```python
from build123d import *

# Parameters (mm, degrees)
SKETCH_1_W          = 15
SKETCH_1_H          = 15
SKETCH_1_W_2        = 13
SKETCH_1_H_2        = 13
EXTRUDE_1_DEPTH     = 37
SKETCH_2_R          = 1.45
CUT_EXTRUDE_1_DEPTH = 41.623269194
SKETCH_3_R          = 1.45
CUT_EXTRUDE_2_DEPTH = 41.623269194


with BuildPart() as part:
    # 草图1 → 凸台-拉伸1 (new body)
    with BuildSketch(Plane(origin=(0, 0, 0), x_dir=(0, 0, -1), z_dir=(1, 0, 0))):
        Rectangle(SKETCH_1_W, SKETCH_1_H)
        Rectangle(SKETCH_1_W_2, SKETCH_1_H_2, mode=Mode.SUBTRACT)
    extrude(amount=EXTRUDE_1_DEPTH)

    # 草图2 → 切除-拉伸1 (cut, through all)
    with BuildSketch(Plane(origin=(0, 0, -7.5), x_dir=(-1, 0, 0), z_dir=(0, 0, -1))):
        with Locations((-11, 0)):
            Circle(SKETCH_2_R)
        with Locations((-26, 0)):
            Circle(SKETCH_2_R)
    extrude(amount=-CUT_EXTRUDE_1_DEPTH, mode=Mode.SUBTRACT)

    # 草图3 → 切除-拉伸2 (cut, through all)
    with BuildSketch(Plane(origin=(0, 7.5, 0), x_dir=(1, 0, 0), z_dir=(0, 1, 0))):
        with Locations(Location((10, 0, 0), (0, 0, 270))):
            Circle(SKETCH_3_R)
        with Locations(Location((30, 0, 0), (0, 0, 270))):
            Circle(SKETCH_3_R)
        with Locations(Location((20, 0, 0), (0, 0, 270))):
            Circle(SKETCH_3_R)
    extrude(amount=-CUT_EXTRUDE_2_DEPTH, mode=Mode.SUBTRACT)


solid = part.part
```
Geometry check sheet. Reference: the model listing, model coordinates, mm. A direction names the side the tool comes from. Give positions to 0.01 mm unless a question says otherwise; leave off trailing zeros. Write each loop counter-clockwise with the first axis right and the second up, starting at its lowest first coordinate (ties: lowest second). Pieces come first, ordered by that corner, then holes.
1) Section check C-C, the plane x = 10. Record the boundary of the cut face in (y, z).
2) Material ranges on L1, parallel to X at y = 7.05, z = 0; L2, parallel to Z at x = 26, y = 2.75, recorded low to high.
3) Section check B-B, the plane x = 26. Record the boundary of the cut face in (y, z), and give its area (3 significant figures).
4) Section check D-D, the plane y = -2. Record the boundary of the cut face in (x, z).
5) Access from +Z, -Z, +X, -X, +Y, -Y to the whole of each face (thin tool, end or side, straight path). Record for faces 4 (the flat face through (18, 6.5, 0)), 5 (the cylindrical face through (24.62, 0.44, -7.01)).
6) Release check for a two-part mould opening along Y. For faces 1 (the cylindrical face through (24.62, 0.44, 6.99)), 2 (the flat face through (18, 0, 7.5)), 3 (the flat face through (18, 7.5, 0)) record: pulls with the +Y half, pulls with the -Y half, needs draft (parallel to the pull), parting line crosses it, or undercut.
7) Section check A-A, the plane z = -1. State how many separate pieces and enclosed holes the cut face has, and give its area (3 significant figures).
Computed:
1. outline: (-7.5, -7.5) - (-1.05, -7.5) - (-1.05, -6.5) - (-6.5, -6.5) - (-6.5, -1.45) - (-7.5, -1.45) - close; (-7.5, 1.45) - (-6.5, 1.45) - (-6.5, 6.5) - (-1.05, 6.5) - (-1.05, 7.5) - (-7.5, 7.5) - close; (1.05, -7.5) - (7.5, -7.5) - (7.5, -1.45) - (6.5, -1.45) - (6.5, -6.5) - (1.05, -6.5) - close; (1.05, 6.5) - (6.5, 6.5) - (6.5, 1.45) - (7.5, 1.45) - (7.5, 7.5) - (1.05, 7.5) - close
2. L1: x = 0 to 8.55, 11.45 to 18.55, 21.45 to 28.55, 31.45 to 37
2. L2: z = -7.5 to -6.5, 6.5 to 7.5
3. outline: (-7.5, -7.5) - (-1.45, -7.5) - (-1.45, -6.5) - (-6.5, -6.5) - (-6.5, 6.5) - (-1.45, 6.5) - (-1.45, 7.5) - (-7.5, 7.5) - close; (1.45, -7.5) - (7.5, -7.5) - (7.5, 7.5) - (1.45, 7.5) - (1.45, 6.5) - (6.5, 6.5) - (6.5, -6.5) - (1.45, -6.5) - close
3. area: 50.2 mm2
4. outline: (0, -7.5) - (37, -7.5) - (37, -6.5) - (0, -6.5) - close; (0, 6.5) - (37, 6.5) - (37, 7.5) - (0, 7.5) - close
5. face 4: +X, -X
5. face 5: +Z, -Z
6. face 1: undercut
6. face 2: needs draft
6. face 3: pulls with the +Y half
7. separate pieces: 8
7. enclosed holes: 0
7. area: 61.4 mm2
